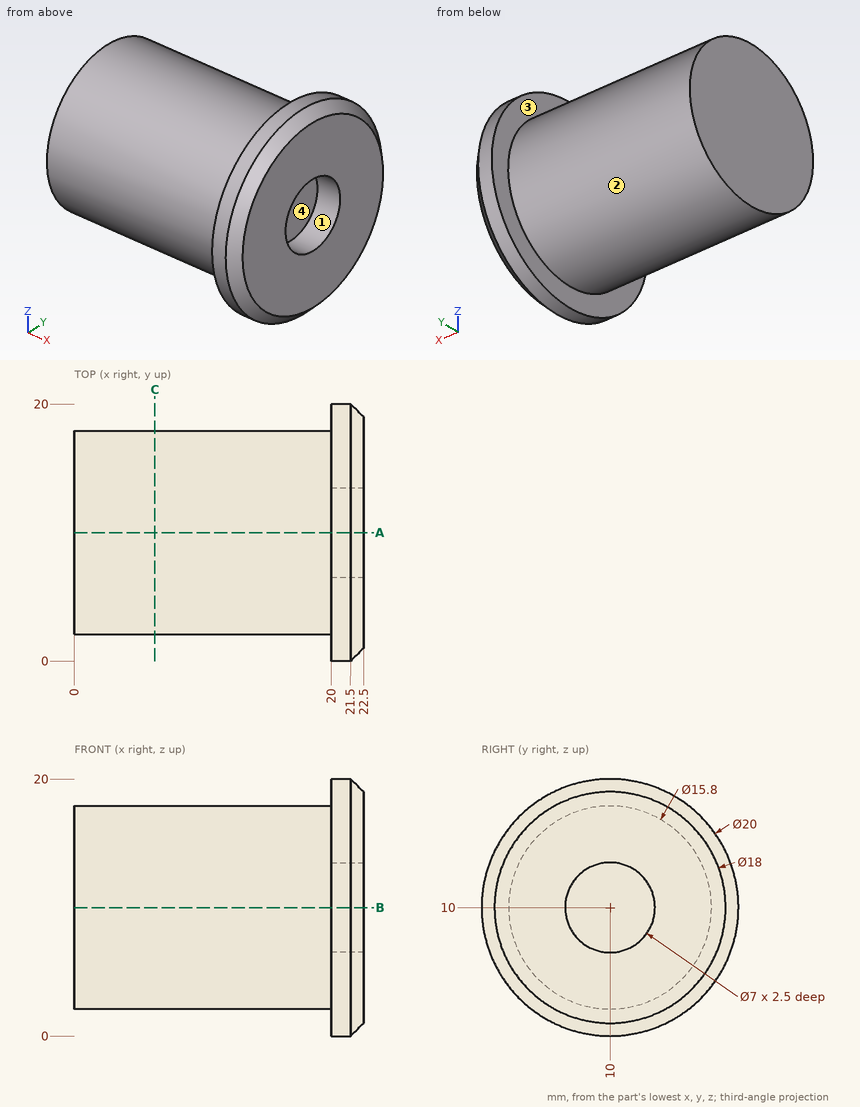
Check sheet for the drawn part. Datum: minimum x, y, z corner. Units: mm. Give positions to 0.01 mm unless a question says otherwise; leave off trailing zeros. Order: outer loops, then holes, each group sorted by start corner. A loop starts at its lowest first (then second) coordinate and runs counter-clockwise, first axis right, second up. Notation, with made-up numbers: (15, 45.25) -> (39, 45.25) arc R19 cw to (39, 73.25) -> close; hole circle Ø1 at (-35.5, 48). An arc over 180 degrees is marked (long way). One line per item, written item: value.
(1) Gauge pin test, flat ends, axial feed: pin 1 (10 mm diameter, centred on x = 5.5, z = 18, fed in from -Y); pin 2 (6 mm diameter, centred on x = 9, z = 15, fed in from -Y); pin 3 (2 mm diameter, centred on x = 4.5, z = 4.5, fed in from +Y). Record the tip position at first contact, or that the pin passes through.
Final values:
pin 1: y = 2.69
pin 2: y = 2.36
pin 3: y = 16.49
(2) Scan lines: line 1 along Y through (x, z) = (21.4, 10); line 2 along X through (y, z) = (2.5, 14.25); line 3 along Y through (x, z) = (21.55, 10). Record each from-to range of solid material in increasing order. Write a range as [from, to].
Final values:
line 1: [0, 6.5], [13.5, 20]
line 2: [20, 22.5]
line 3: [0.05, 6.5], [13.5, 19.95]
(3) Draft check along Y on the marked faces 1, 2, 3 and 4. Enter one of: pulls with the +Y half, pulls with the -Y half, needs draft (parallel to the pull), parting line crosses it, or undercut.
Final values:
face 1: undercut
face 2: parting line crosses it
face 3: needs draft
face 4: undercut
(4) Sectioned sample at C-C on x = 6.25. Record the cut outline in (y, z), then the cut area to 3 significant figures.
Final values:
outline: circle Ø15.8 at (10, 10)
area: 196 mm^2
(5) Sectioned sample at A-A on y = 10. Record the cut outline in (x, z).
Final values:
outline: (0, 2.1) -> (20, 2.1) -> (20, 0) -> (21.5, 0) -> (22.5, 1) -> (22.5, 6.5) -> (20, 6.5) -> (20, 13.5) -> (22.5, 13.5) -> (22.5, 19) -> (21.5, 20) -> (20, 20) -> (20, 17.9) -> (0, 17.9) -> close
